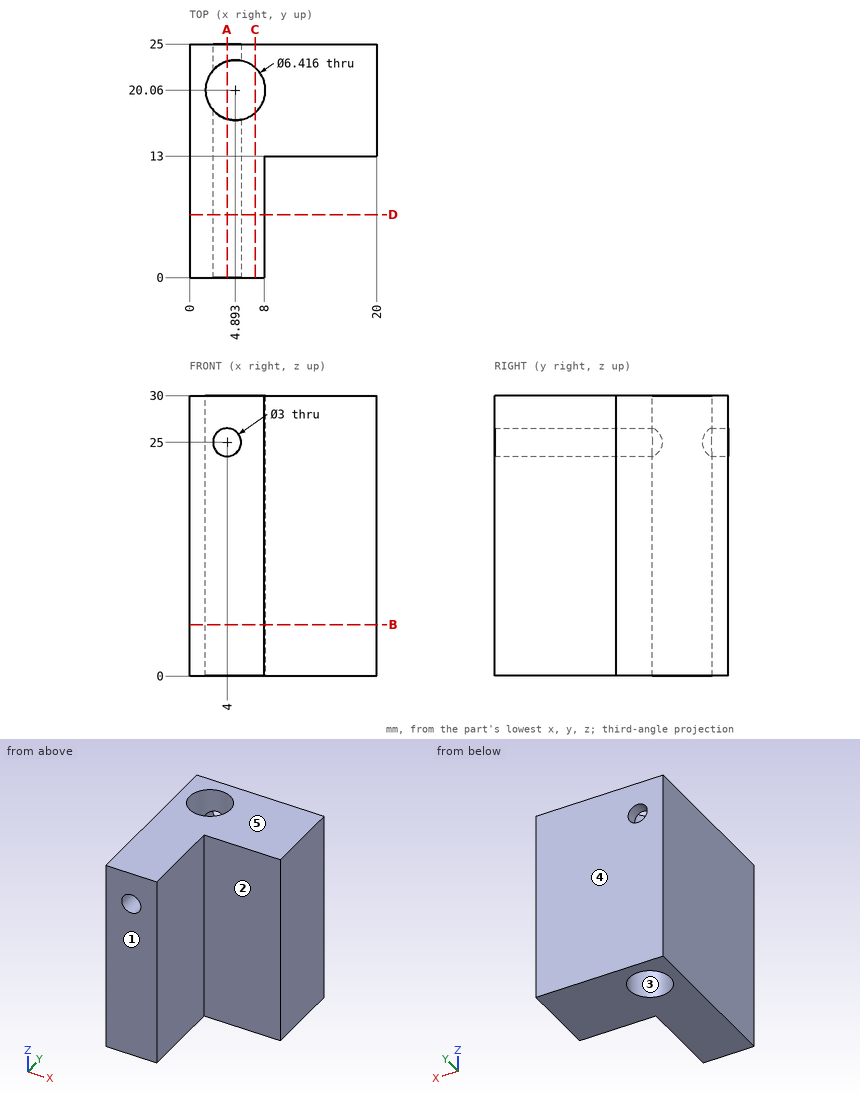
Here's the drawing with two shaded views (mm, measured from the low corner). I have some questions. A direction names the side the tool comes from. Give positions to 0.01 mm unless a question says otherwise; leave off trailing zeros. Loops run counter-clockwise (first coordinate to the right, second up) from the corner with the lowest first, then second, coordinate; pieces in that order, holes last. Notation, with made-up numbers: (3, 33) -> (30, 33) arc R14 ccw to (30, 49) -> close; hole circle Ø8 at (73, -12). An arc over 180 degrees is marked (long way). Use one line per item in the form item = value.
1) I need wall thicknesses on line 1 along Z through (x, y) = (4, 9.25); line 2 along X through (y, z) = (3, 14); line 3 along Y through (x, z) = (10.75, 12.5). Which ranges of each line are inside material? Lowest first, please.
Answers:
line_1 = 0 to 23.5, 26.5 to 30
line_2 = 0 to 8
line_3 = 13 to 25
2) Will these pins go through, and if not, where does the flat tip stop? pin 1 (3 mm diameter, centred on x = 15, z = 5, fed in from -Y); pin 2 (2.5 mm diameter, centred on x = 4, z = 25, fed in from +Y); pin 3 (14.5 mm diameter, centred on y = 5, z = 9, fed in from +X).
Answers:
pin_1 = 13
pin_2 = through
pin_3 = 8
3) If we section it at C-C (x = 7): Please give me the cut outline in (y, z), plus the area to 3 significant figures.
Answers:
outline = (0, 0) -> (17.64, 0) -> (17.64, 30) -> (0, 30) -> close; (22.48, 0) -> (25, 0) -> (25, 30) -> (22.48, 30) -> close
area = 605 mm²
4) For the marked faces 1 and 2, which set-ups out of +Z, -Z, +X, -X, +Y, -Y let a thin tool reach every point of the face, with its end or its side?
Answers:
face_1 = +Z, -Z, +X, -X, -Y
face_2 = +Z, -Z, +X, -Y
5) If we section it at B-B (z = 5.5): Please give me the cut outline in (x, y), plus the area to 3 significant figures.
Answers:
outline = (0, 0) -> (8, 0) -> (8, 13) -> (20, 13) -> (20, 25) -> (0, 25) -> close; hole circle Ø6.42 at (4.89, 20.06)
area = 312 mm²
6) We'd pull the mould along Y, two halves only. Please class the marked faces 3, 4 and 5: released by +Y, released by -Y, zero draft, split by the parting line, or undercut.
Answers:
face_3 = undercut
face_4 = released by +Y
face_5 = zero draft
7) If we section it at A-A (x = 4): Please give me the cut outline in (y, z).
Answers:
outline = (0, 0) -> (16.98, 0) -> (16.98, 23.5) -> (0, 23.5) -> close; (0, 26.5) -> (16.98, 26.5) -> (16.98, 30) -> (0, 30) -> close; (23.14, 0) -> (25, 0) -> (25, 23.5) -> (23.14, 23.5) -> close; (23.14, 26.5) -> (25, 26.5) -> (25, 30) -> (23.14, 30) -> close
8) If we section it at D-D (y = 6.75): Please give me the cut outline in (x, z).
Answers:
outline = (0, 0) -> (8, 0) -> (8, 30) -> (0, 30) -> close; hole circle Ø3 at (4, 25)
